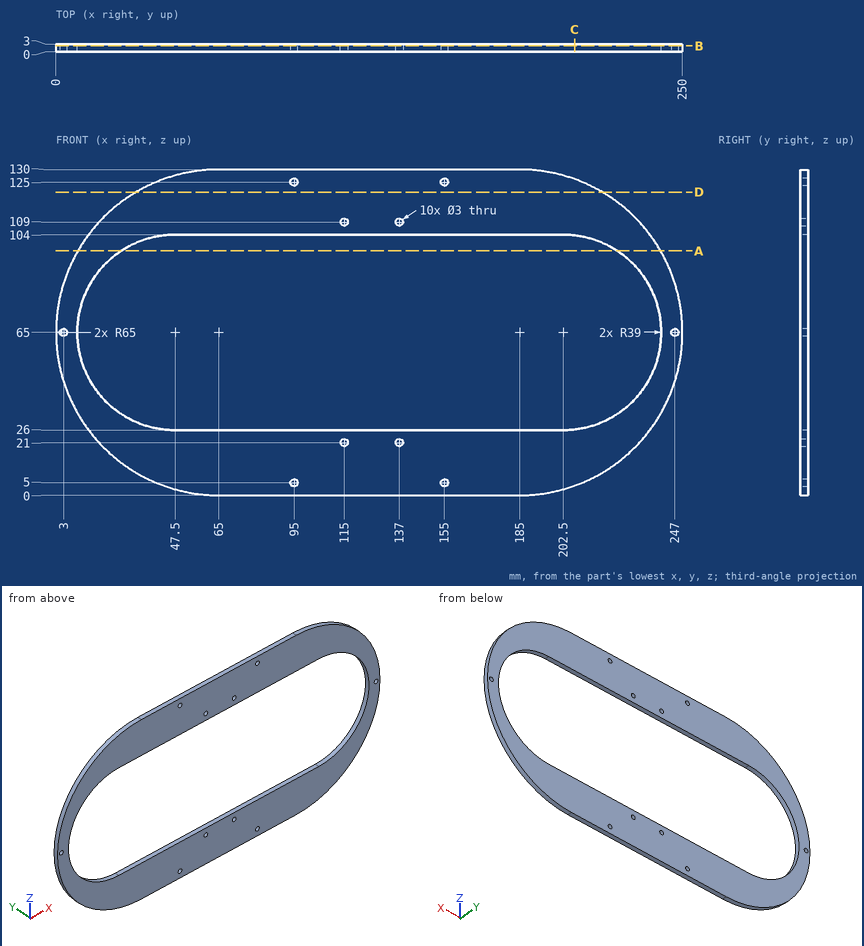
For this review, use the dimensioned drawing (mm, ordinates from the lowest corner) and the shaded views. Round coordinates to 2 decimals unless told otherwise and drop trailing zeros. Write each loop counter-clockwise with the first axis right and the second up, starting at its lowest first coordinate (ties: lowest second). Pieces come first, ordered by that corner, then holes. Notation, with made-up numbers: M 73,77 L 132,77 A16 cw 132,102 Z; hole C 33,25.25 d10. An arc over 180 degrees is marked long. Write item = value, one per line. Start each with the question number.
(1) We need section C-C (x = 207). Give the boundary of the cut face in (y, z), then the cut area to 3 significant figures.
(2) We need section D-D (z = 121). Give the boundary of the cut face in (x, y), then the cut area to 3 significant figures.
(3) We need section B-B (y = 2.3). Give the number of separate pieces and of enclosed holes in the cut face, then the cut area to 3 significant figures.
(4) We need section A-A (z = 97.5). Give the boundary of the cut face in (x, y).
(5) For line 1 along Z through (x, y) = (137, 0.8); line 2 along Z through (x, y) = (95, 2.35); line 3 along Z through (x, y) = (187, 0.85), list the stretches that pass through material, from the lowest coordinate up.
Results found:
q1.outline = M 0,3.84 L 3,3.84 L 3,26.26 L 0,26.26 Z; M 0,103.74 L 3,103.74 L 3,126.16 L 0,126.16 Z
q1.area = 135 mm²
q2.outline = M 32,0 L 218,0 L 218,3 L 32,3 Z
q2.area = 558 mm²
q3.separate_pieces = 1
q3.enclosed_holes = 11
q3.area = 11,900 mm²
q4.outline = M 8.71,0 L 25.94,0 L 25.94,3 L 8.71,3 Z; M 224.06,0 L 241.29,0 L 241.29,3 L 224.06,3 Z
q5.line_1 = 0 to 19.5, 22.5 to 26, 104 to 107.5, 110.5 to 130
q5.line_2 = 0 to 3.5, 6.5 to 26, 104 to 123.5, 126.5 to 130
q5.line_3 = 0.03 to 26, 104 to 129.97
